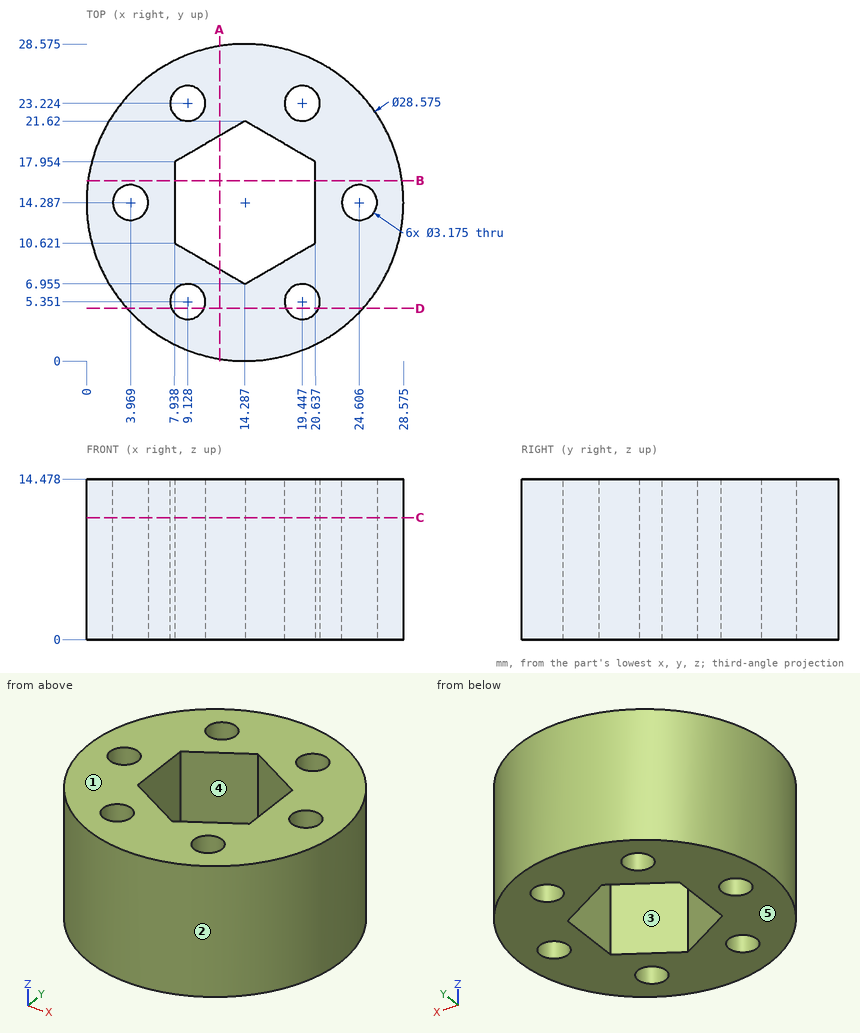
The figure shows three views and two pictorial views of one solid part (mm, origin at its lowest corner). Answer the questions. A direction names the side the tool comes from. Coordinates: 2 decimals unless noted, no trailing zeros. Loops run counter-clockwise (first coordinate to the right, second up) from the corner with the lowest first, then second, coordinate; pieces in that order, holes last. Notation, with made-up numbers: M 68.5,81 L 127.5,81 A19 cw 127.5,96 Z; hole C 57.25,-30.75 d5. An arc over 180 degrees is marked long. Use CSV: the item, a comma, the result in double quotes. Start each with the question number.
(1) Find section D-D, the plane y = 4.75. State how many separate pieces and enclosed holes the cut face has, then the cut area to 3 significant figures.
(2) Consider line 1 (Y direction, x = 8, z = 9.5) (1 decimal); line 2 (Y direction, x = 17, z = 13.75) (1 decimal); line 3 (Y direction, x = 13.5, z = 0.75) (1 decimal). Determine where each line is inside the solid, lowest interval first.
(3) Find section A-A, the plane x = 12. Give the vertices of the cut face in (y, z) (1 decimal).
(4) For a pull along X with two mould halves and no side action, classify the marked faces 1, 2 and 3 as +X half, -X half, draft (parallel to the pull), parting line (faces both ways), or undercut.
(5) For the marked faces 4 and 5, determine the directions among +Z, -Z, +X, -X, +Y, -Y from which every point of the face is accessible in a straight line to the end or side of a thin tool.
(6) Given pin 1 Ø2 at (y, z) = (12.5, 9.5) entering from -X; pin 2 Ø4 at (y, z) = (3.5, 6.5) entering from +X; pin 3 Ø5 at (x, z) = (7, 6.5) entering from -Y (1 decimal), each flat-ended and moving along its own axis, determine where each tip first touches the part or whether it passes through.
(7) Find section C-C, the plane z = 11. Give the vertices of the cut face in (x, y) (1 decimal).
(8) Find section B-B, the plane y = 16.25. Give the vertices of the cut face in (x, z) (1 decimal).
Recorded:
1,separate pieces,"3"
1,enclosed holes,"0"
1,area,"223 mm^2"
2,line 1,"y = 1.5 to 4.2, 6.5 to 10.6, 18 to 22.1, 24.3 to 27.1"
2,line 2,"y = 0.3 to 8.5, 20.1 to 28.3"
2,line 3,"y = 0 to 7.4, 21.2 to 28.6"
3,outline,"M 0.2,0 L 8.3,0 L 8.3,14.5 L 0.2,14.5 Z; M 20.3,0 L 28.4,0 L 28.4,14.5 L 20.3,14.5 Z"
4,face 1,"draft"
4,face 2,"parting line"
4,face 3,"undercut"
5,face 4,"+Z, -Z"
5,face 5,"-Z, +X, -X, +Y, -Y"
6,pin 1,"stops at x = 0.02"
6,pin 2,"stops at x = 25.55"
6,pin 3,"stops at y = 0.8"
7,outline,"C 14.3,14.3 d28.6; hole C 4,14.3 d3.2; hole C 9.1,5.4 d3.2; hole C 9.1,23.2 d3.2; hole M 7.9,10.6 L 14.3,7 L 20.6,10.6 L 20.6,18 L 14.3,21.6 L 7.9,18 Z; hole C 19.4,5.4 d3.2; hole C 19.4,23.2 d3.2; hole C 24.6,14.3 d3.2"
8,outline,"M 0.1,0 L 7.9,0 L 7.9,14.5 L 0.1,14.5 Z; M 20.6,0 L 28.4,0 L 28.4,14.5 L 20.6,14.5 Z"
